Design review of the part built by this model. Coordinates are the model's own, in mm. Give positions to 0.01 mm unless a question says otherwise; leave off trailing zeros. Loops run counter-clockwise (first coordinate to the right, second up) from the corner with the lowest first, then second, coordinate; pieces in that order, holes last. Notation, with made-up numbers: (-4, 58) -> (42, 58) arc R20 cw to (42, 84) -> close; hole circle Ø7 at (-10.5, -29.75). An arc over 180 degrees is marked (long way). Answer in a Markdown table with one row per item. Add a question column.
(1) Draft analysis for pull direction Z (two halves, no side actions). For faces 1 (the flat face through (-9, 0.8, -10)), 2 (the cylindrical face through (-0.764, 0.406, -0.724)), 3 (the cylindrical face through (-1.53, 0.39, -1.77)), state which applies: +Z half, -Z half, draft (parallel to the pull), parting line (faces both ways), or undercut.
(2) Consider section A-A on y = 0.2. Write out the cut boundary in (x, z).
(3) For line 1 (Z direction, x = -16.51, y = 0.2); line 2 (Z direction, x = -18, y = 0.65), list the stretches that pass through material, from the lowest coordinate up.
(4) Consider section C-C on z = -18.5. Write out the cut boundary in (x, y), then the cut area to 3 significant figures.
(5) Consider section B-B on x = -1.75. Write out the cut boundary in (y, z).
Autodesk Inventor part; units mm, degrees
ref_plane "YZ Plane" through (0, 0, 0) normal (1, 0, 0) x (0, 1, 0)
ref_plane "XZ Plane" through (0, 0, 0) normal (0, 1, 0) x (-1, 0, 0)
ref_plane "XY Plane" through (0, 0, 0) normal (0, 0, 1) x (1, 0, 0)
sketch "Sketch1" plane through (0, 0, 0) normal (0, 1, 0) x (-1, 0, 0)
  line L0 (0, 0) -> (19.05, 0)
  line L1 (19.05, 0) -> (19.05, -20.32)
  line L2 (19.05, -20.32) -> (0, -20.32)
  line L3 (0, -20.32) -> (0, 0)
  circle A0 centre (16.51, -2.54) radius 1.2639
  circle A1 centre (16.51, -17.78) radius 1.27
  circle A2 centre (2.54, -17.78) radius 1.27
  circle A3 centre (2.54, -2.54) radius 1.27
  dimension "d0" = 20.32
  dimension "d1" = 19.05
  dimension "d2" = 15.24
  dimension "d3" = 2.54
  dimension "d4" = 15.24
  dimension "d5" = 13.97
  dimension "d6" = 2.54
  dimension "d7" = 13.97
  dimension "d8" = 2.54
  dimension "d9" = 2.54
  dimension "d10" = 2.54
  dimension "d11" = 2.54
  dimension "d12" = 2.54
  dimension "d13" = 2.54
extrude "Extrusion1" add sketch "Sketch1" along normal blind 0.8
fillet "Fillet1" radius 2.54 4 edges at (0, 0.4, 0) (0, 0.4, -20.32) (-19.05, 0.4, -20.32) (-19.05, 0.4, 0)
properties part number "micro lipo footprint"
Values follow:
| question | item | result |
|---|---|---|
| 1 | face 1 | draft |
| 1 | face 2 | +Z half |
| 1 | face 3 | undercut |
| 2 | outline | (-19.05, -17.78) arc R2.54 ccw to (-16.51, -20.32) -> (-2.54, -20.32) arc R2.54 ccw to (0, -17.78) -> (0, -2.54) arc R2.54 ccw to (-2.54, 0) -> (-16.51, 0) arc R2.54 ccw to (-19.05, -2.54) -> close; hole circle Ø2.54 at (-16.51, -17.78); hole circle Ø2.53 at (-16.51, -2.54); hole circle Ø2.54 at (-2.54, -17.78); hole circle Ø2.54 at (-2.54, -2.54) |
| 3 | line 1 | -20.32 to -19.05, -16.51 to -3.8, -1.28 to 0 |
| 3 | line 2 | -19.84 to -0.48 |
| 4 | outline | (-18.95, 0) -> (-17.56, 0) -> (-17.56, 0.8) -> (-18.95, 0.8) -> close; (-15.46, 0) -> (-3.59, 0) -> (-3.59, 0.8) -> (-15.46, 0.8) -> close; (-1.49, 0) -> (-0.1, 0) -> (-0.1, 0.8) -> (-1.49, 0.8) -> close |
| 4 | area | 11.7 mm2 |
| 5 | outline | (0, -20.19) -> (0.8, -20.19) -> (0.8, -18.77) -> (0, -18.77) -> close; (0, -16.79) -> (0.8, -16.79) -> (0.8, -3.53) -> (0, -3.53) -> close; (0, -1.55) -> (0.8, -1.55) -> (0.8, -0.13) -> (0, -0.13) -> close |
